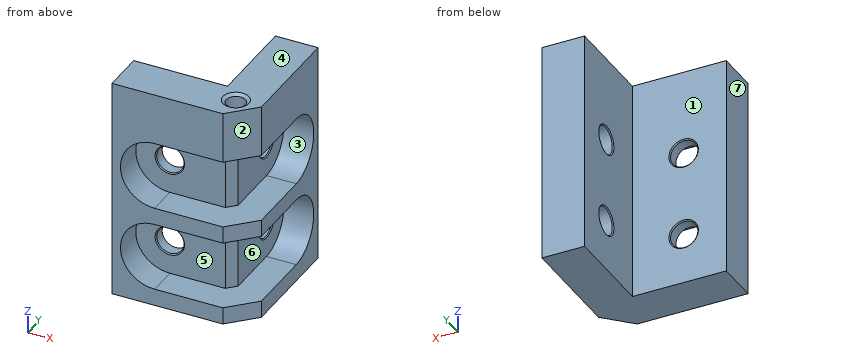
```python
from build123d import *

# Parameters (mm, degrees)
SKETCH_1_W                    = 16
SKETCH_1_H                    = 16
EXTRUDE_1_DEPTH               = 26
CUT_EXTRUDE_1_DEPTH           = 29.354893758
CUT_EXTRUDE_2_DEPTH           = 3.5
CUT_EXTRUDE_3_DEPTH           = 3.5
CHAMFER_1_SIZE                = 1
HOLE_WIZARD_4_401_D           = 2.2606
HOLE_WIZARD_4_401_DEPTH       = 6
HOLE_WIZARD_4_401_CSINK_D     = 3.048
HOLE_WIZARD_4_401_CSINK_ANGLE = 110
CHAMFER_3_SIZE                = 3


with BuildPart() as part:
    # Эскиз1 → Вытянуть1 (new body)
    with BuildSketch(Plane.XY):
        Rectangle(SKETCH_1_W, SKETCH_1_H)
    extrude(amount=EXTRUDE_1_DEPTH)

    # Эскиз2 → Вырез-Вытянуть1 (cut, through all)
    with BuildSketch(Plane(origin=(0, 0, 0), x_dir=(-1, 0, 0), z_dir=(0, 0, -1))):
        Polygon((-3, 56.832975678), (-3, 8), (-3, -3), (8, -3), (56.832975678, -3), (125.893232173, 66.060256495), (66.060256495, 125.893232173), align=None)
    extrude(amount=-CUT_EXTRUDE_1_DEPTH, mode=Mode.SUBTRACT)

    # Эскиз9 → Вырез-Вытянуть2 (cut)
    with BuildSketch(Plane(origin=(8, 0, 0), x_dir=(0, 0, -1), z_dir=(1, 0, 0))):
        with BuildLine():
            Line((-20, 3), (-20, -8))
            Line((-20, -8), (-12, -8))
            Line((-12, -8), (-12, 3))
            ThreePointArc((-12, 3), (-16, 7), (-20, 3))
        make_face()
        with BuildLine():
            Line((-10, 3), (-10, -8))
            Line((-10, -8), (-2, -8))
            Line((-2, -8), (-2, 3))
            ThreePointArc((-2, 3), (-6, 7), (-10, 3))
        make_face()
    extrude(amount=-CUT_EXTRUDE_2_DEPTH, mode=Mode.SUBTRACT)

    # Эскиз10 → Вырез-Вытянуть3 (cut)
    with BuildSketch(Plane.XZ.offset(8)):
        with BuildLine():
            Line((4.5, 20), (-3, 20))
            ThreePointArc((-3, 20), (-7, 16), (-3, 12))
            Line((-3, 12), (4.5, 12))
            Line((4.5, 12), (4.5, 20))
        make_face()
        with BuildLine():
            Line((4.5, 10), (-3, 10))
            ThreePointArc((-3, 10), (-7, 6), (-3, 2))
            Line((-3, 2), (4.5, 2))
            Line((4.5, 2), (4.5, 10))
        make_face()
    extrude(amount=-CUT_EXTRUDE_3_DEPTH, mode=Mode.SUBTRACT)

    # Фаска1
    chamfer_1_edges = [part.edges().sort_by_distance(p)[0] for p in [
        (4.5, -4.5, 16),
        (4.5, -4.5, 6),
    ]]
    chamfer(chamfer_1_edges, length=CHAMFER_1_SIZE)

    # Отверстие обработанное метчиком #4-401
    with Locations(Plane(origin=(-3.054370164, -0.984217205, 26), x_dir=(-1, 0, 0), z_dir=(0, 0, 1))):
        with Locations((-8.054370164, 4.015782795)):
            CounterSinkHole(HOLE_WIZARD_4_401_D / 2, HOLE_WIZARD_4_401_CSINK_D / 2, depth=HOLE_WIZARD_4_401_DEPTH, counter_sink_angle=HOLE_WIZARD_4_401_CSINK_ANGLE)

    # Эскиз11 → Отверстие с зазором M31 (revolve, cut)
    with BuildSketch(Plane(origin=(-3, -4.5, 16), x_dir=(0, 0, -1), z_dir=(1, 0, 0))):
        Polygon((0, 0), (0, 1.5), (1.725, 1.5), (1.6, 1.375), (1.6, 0.125), (1.725, 0), align=None)
    revolve(axis=Axis((-3, -10.85, 16), (0, 1, 0)), mode=Mode.SUBTRACT)

    # Эскиз11 at point 2 (carried to point 2, square into its face) → Отверстие с зазором M31 at 2 (revolve, cut)
    with BuildSketch(Plane(origin=(-3, -4.5, 6), x_dir=(0, 0, -1), z_dir=(1, 0, 0))):
        Polygon((0, 0), (0, 1.5), (1.725, 1.5), (1.6, 1.375), (1.6, 0.125), (1.725, 0), align=None)
    revolve(axis=Axis((-3, -10.85, 6), (0, 1, 0)), mode=Mode.SUBTRACT)

    # Эскиз11 at point 3 (carried to point 3, square into its face) → Отверстие с зазором M31 at 3 (revolve, cut)
    with BuildSketch(Plane(origin=(4.5, 3, 6), x_dir=(0, 0, -1), z_dir=(0, 1, 0))):
        Polygon((0, 0), (0, 1.5), (1.725, 1.5), (1.6, 1.375), (1.6, 0.125), (1.725, 0), align=None)
    revolve(axis=Axis((10.85, 3, 6), (-1, 0, 0)), mode=Mode.SUBTRACT)

    # Эскиз11 at point 4 (carried to point 4, square into its face) → Отверстие с зазором M31 at 4 (revolve, cut)
    with BuildSketch(Plane(origin=(4.5, 3, 16), x_dir=(0, 0, -1), z_dir=(0, 1, 0))):
        Polygon((0, 0), (0, 1.5), (1.725, 1.5), (1.6, 1.375), (1.6, 0.125), (1.725, 0), align=None)
    revolve(axis=Axis((10.85, 3, 16), (-1, 0, 0)), mode=Mode.SUBTRACT)

    # Фаска3
    chamfer_3_edges = [part.edges().sort_by_distance(p)[0] for p in [
        (8, -8, 11),
        (8, -8, 1),
        (8, -8, 23),
    ]]
    chamfer(chamfer_3_edges, length=CHAMFER_3_SIZE)


solid = part.part
```
Geometry check sheet. Reference: the model listing, model coordinates, mm. Face numbers are marked on the shaded views. A direction names the side the tool comes from. Coordinates: 2 decimals unless noted, no trailing zeros. Order: outer loops, then holes, each group sorted by start corner. A loop starts at its lowest first (then second) coordinate and runs counter-clockwise, first axis right, second up. Notation, with made-up numbers: (-5.75, 4) - (41.25, 4) arc R36 cw to (41.25, 38) - close; hole circle Ø1 at (-23, 60). An arc over 180 degrees is marked (long way). Answer as a JSON object with one key per item and string values. Group by question number.
Item 1: Scan lines: probe 1 along Z at (x, y) = (6.75, -2.75); probe 2 along Z at (x, y) = (4, 3); probe 3 along X at (y, z) = (-3.4, 6). Record each from-to range of solid material in increasing order.
Item 2: Draft check along Z on the marked faces 4, 5, 6 and 7. Enter one of: +Z half, -Z half, draft (parallel to the pull), parting line (faces both ways), or undercut.
Item 3: Depth check by flat-ended pin: pin 1 Ø4 at (x, z) = (-4, 4.5) entering from -Y; pin 2 Ø9 at (x, z) = (-4, 15.5) entering from +Y; pin 3 Ø3 at (y, z) = (1, 13) entering from -X. Enter the tip coordinate at first touch or a pass-through.
Item 4: Sectioned sample at D-D, the plane y = -0.75. Record the cut outline in (x, z), and give its area (3 significant figures).
Item 5: Sectioned sample at B-B, the plane z = 20.75. Record the cut outline in (x, y), and give its area (3 significant figures).
Item 6: Tool access check on the marked faces 1, 2 and 3. Record the directions out of +Z, -Z, +X, -X, +Y, -Y that give a thin tool (end or side, any length) a straight path to the whole face; none if there is none.
Item 7: Sectioned sample at C-C, the plane x = 0.75. Record the cut outline in (y, z).
Item 8: Sectioned sample at A-A, the plane z = 16. Record the cut outline in (x, y) (3 decimals).
Resolved:
{
 "1": {"probe 1": "0 to 2, 10 to 12, 20 to 26", "probe 2": "0 to 4.4, 7.6 to 14.4, 17.6 to 26", "probe 3": "-8 to -4.6, -1.4 to 4.5"},
 "2": {"face 4": "+Z half", "face 5": "undercut", "face 6": "undercut", "face 7": "draft"},
 "3": {"pin 1": "y = -4.5", "pin 2": "y = -3", "pin 3": "x = 3"},
 "4": {"outline": "(3, 0) - (8, 0) - (8, 2) - (4.5, 2) - (4.5, 10) - (8, 10) - (8, 12) - (4.5, 12) - (4.5, 20) - (8, 20) - (8, 26) - (3, 26) - close", "area": "74.0 mm^2"},
 "5": {"outline": "(-8, -8) - (5, -8) - (8, -5) - (8, 8) - (3, 8) - (3, -3) - (-8, -3) - close; hole circle Ø2.26 at (5, -5)", "area": "126 mm^2"},
 "6": {"face 1": "+Z, -Z, -X, +Y", "face 2": "+Z, -Z, +X, -Y", "face 3": "+X, -Y"},
 "7": {"outline": "(-8, 0) - (-3, 0) - (-3, 26) - (-8, 26) - (-8, 20) - (-4.5, 20) - (-4.5, 12) - (-8, 12) - (-8, 10) - (-4.5, 10) - (-4.5, 2) - (-8, 2) - close"},
 "8": {"outline": "(-8, -8) - (-7, -8) - (-7, -4.5) - (-4.725, -4.5) - (-4.6, -4.375) - (-4.6, -3.125) - (-4.725, -3) - (-8, -3) - close; (-1.4, -4.375) - (-1.275, -4.5) - (3.5, -4.5) - (4.5, -3.5) - (4.5, 1.275) - (4.375, 1.4) - (3.125, 1.4) - (3, 1.275) - (3, -3) - (-1.275, -3) - (-1.4, -3.125) - close; (3, 4.725) - (3.125, 4.6) - (4.375, 4.6) - (4.5, 4.725) - (4.5, 7) - (8, 7) - (8, 8) - (3, 8) - close"}
}
